Geometry check sheet. Reference: drawing and pictorial views, mm from the part's lowest x, y, z. A direction names the side the tool comes from. Round coordinates to 2 decimals unless told otherwise and drop trailing zeros. Write each loop counter-clockwise with the first axis right and the second up, starting at its lowest first coordinate (ties: lowest second). Pieces come first, ordered by that corner, then holes. Notation, with made-up numbers: M 63,-0.5 L 79,-0.5 A25 ccw 79,31.5 Z; hole C 19.5,-22.75 d6. An arc over 180 degrees is marked long. Answer in a Markdown table with one row per item.
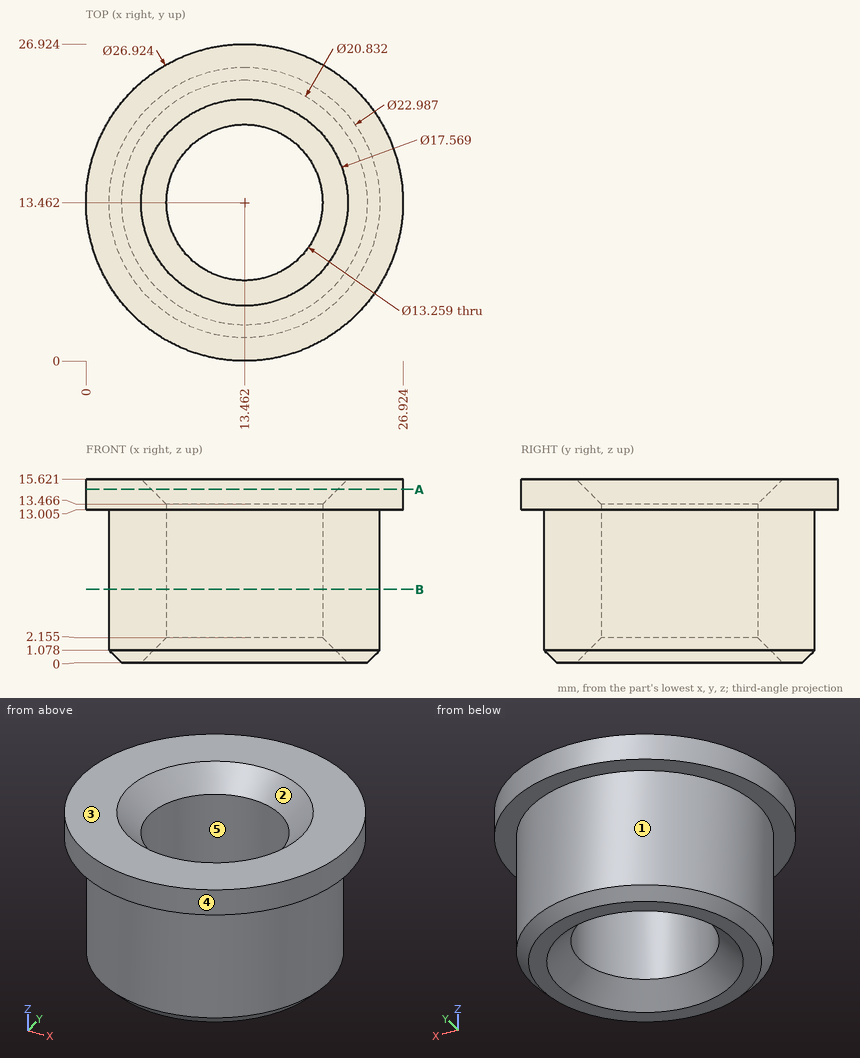
1. Access from +Z, -Z, +X, -X, +Y, -Y to the whole of each face (thin tool, end or side, straight path). Record for the marked faces 1 and 2.
Found:
| item | result |
|---|---|
| face 1 | -Z |
| face 2 | +Z |
2. Draft check along X on the marked faces 3, 4 and 5. Enter one of: +X half, -X half, draft (parallel to the pull), parting line (faces both ways), or undercut.
Found:
| item | result |
|---|---|
| face 3 | draft |
| face 4 | parting line |
| face 5 | undercut |
3. Scan lines: L1, parallel to X at y = 8.5, z = 10.5 (1 decimal); L2, parallel to Y at x = 10.5, z = 15 (1 decimal); L3, parallel to X at y = 17, z = 2.25 (1 decimal). Record each from-to range of solid material in increasing order.
Found:
| item | result |
|---|---|
| L1 | x = 3.1 to 9.1, 17.9 to 23.8 |
| L2 | y = 0.3 to 5.9, 21.1 to 26.6 |
| L3 | x = 2.5 to 7.9, 19.1 to 24.4 |
4. Section check B-B, the plane z = 6.25. Record the cut outline in (x, y) (1 decimal).
Found:
| item | result |
|---|---|
| outline | C 13.5,13.5 d23; hole C 13.5,13.5 d13.3 |
5. Section check A-A, the plane z = 14.75. Record the cut outline in (x, y) (1 decimal).
Found:
| item | result |
|---|---|
| outline | C 13.5,13.5 d26.9; hole C 13.5,13.5 d15.8 |
6. Go/stop test with flat-tipped pins: pin 1 (6 mm diameter, centred on y = 21.5, z = 9.5, fed in from -X); pin 2 (1.5 mm diameter, centred on x = 19.5, z = 9, fed in from +Y); pin 3 (6 mm diameter, centred on x = 10.5, z = 3.5, fed in from +Y). Record where each tip stops, or that it passes through.
Found:
| item | result |
|---|---|
| pin 1 | stops at x = 3.13 |
| pin 2 | stops at y = 23.67 |
| pin 3 | stops at y = 24.96 |
